Check sheet for the modelled part. Datum: model origin and axes. Units: mm. Coordinates: 2 decimals unless noted, no trailing zeros. Use CSV: the item, a comma, the result in double quotes.
```python
from build123d import *

# Parameters (mm, degrees)
SKETCH_1_R          = 1
EXTRUDE_1_DEPTH     = 2
SKETCH_2_R          = 1
CUT_EXTRUDE_1_DEPTH = 10
SKETCH_3_R          = 1.5
CUT_EXTRUDE_2_DEPTH = 10


with BuildPart() as part:
    # 草圖1 → 填料-伸長1 (new body)
    with BuildSketch(Plane.XY):
        with BuildLine():
            Line((23.861531606, 13.243524775), (25.861531606, 13.243524775))
            ThreePointArc((25.861531606, 13.243524775), (26.568638387, 13.536417994), (26.861531606, 14.243524775))
            Line((26.861531606, 14.243524775), (26.861531606, 16.243524775))
            Line((26.861531606, 16.243524775), (80.861531606, 16.243524775))
            Line((80.861531606, 16.243524775), (81.861531606, 16.243524775))
            Line((81.861531606, 16.243524775), (81.861531606, 15.243524775))
            Line((81.861531606, 15.243524775), (81.861531606, -7.006475225))
            Line((81.861531606, -7.006475225), (79.861531606, -7.006475225))
            ThreePointArc((79.861531606, -7.006475225), (79.154424825, -7.299368444), (78.861531606, -8.006475225))
            Line((78.861531606, -8.006475225), (78.861531606, -10.006475225))
            ThreePointArc((78.861531606, -10.006475225), (79.154424825, -10.713582006), (79.861531606, -11.006475225))
            Line((79.861531606, -11.006475225), (81.861531606, -11.006475225))
            Line((81.861531606, -11.006475225), (81.861531606, -39.006475225))
            Line((81.861531606, -39.006475225), (81.861531606, -40.006475225))
            Line((81.861531606, -40.006475225), (80.861531606, -40.006475225))
            Line((80.861531606, -40.006475225), (61.861531606, -40.006475225))
            Line((61.861531606, -40.006475225), (61.861531606, -38.006475225))
            ThreePointArc((61.861531606, -38.006475225), (61.568638387, -37.299368444), (60.861531606, -37.006475225))
            Line((60.861531606, -37.006475225), (58.861531606, -37.006475225))
            ThreePointArc((58.861531606, -37.006475225), (58.154424825, -37.299368444), (57.861531606, -38.006475225))
            Line((57.861531606, -38.006475225), (57.861531606, -40.006475225))
            Line((57.861531606, -40.006475225), (-8.138468394, -40.006475225))
            Line((-8.138468394, -40.006475225), (-8.138468394, -38.006475225))
            ThreePointArc((-8.138468394, -38.006475225), (-8.431361613, -37.299368444), (-9.138468394, -37.006475225))
            Line((-9.138468394, -37.006475225), (-11.138468394, -37.006475225))
            ThreePointArc((-11.138468394, -37.006475225), (-11.845575175, -37.299368444), (-12.138468394, -38.006475225))
            Line((-12.138468394, -38.006475225), (-12.138468394, -40.006475225))
            Line((-12.138468394, -40.006475225), (-31.138468394, -40.006475225))
            Line((-31.138468394, -40.006475225), (-32.138468394, -40.006475225))
            Line((-32.138468394, -40.006475225), (-32.138468394, -39.006475225))
            Line((-32.138468394, -39.006475225), (-32.138468394, -11.006475225))
            Line((-32.138468394, -11.006475225), (-30.138468394, -11.006475225))
            ThreePointArc((-30.138468394, -11.006475225), (-29.431361613, -10.713582006), (-29.138468394, -10.006475225))
            Line((-29.138468394, -10.006475225), (-29.138468394, -8.006475225))
            ThreePointArc((-29.138468394, -8.006475225), (-29.431361613, -7.299368444), (-30.138468394, -7.006475225))
            Line((-30.138468394, -7.006475225), (-32.138468394, -7.006475225))
            Line((-32.138468394, -7.006475225), (-32.138468394, 15.243524775))
            Line((-32.138468394, 15.243524775), (-32.138468394, 16.243524775))
            Line((-32.138468394, 16.243524775), (-31.138468394, 16.243524775))
            Line((-31.138468394, 16.243524775), (22.861531606, 16.243524775))
            Line((22.861531606, 16.243524775), (22.861531606, 14.243524775))
            ThreePointArc((22.861531606, 14.243524775), (23.154424825, 13.536417994), (23.861531606, 13.243524775))
        make_face()
        with Locations((55.861531606, -36.006475225)):
            Circle(SKETCH_1_R, mode=Mode.SUBTRACT)
        with Locations((77.861531606, -5.006475225)):
            Circle(SKETCH_1_R, mode=Mode.SUBTRACT)
        with Locations((-6.138468394, -36.006475225)):
            Circle(SKETCH_1_R, mode=Mode.SUBTRACT)
        with Locations((28.861531606, 12.243524775)):
            Circle(SKETCH_1_R, mode=Mode.SUBTRACT)
        with Locations((20.861531606, 12.243524775)):
            Circle(SKETCH_1_R, mode=Mode.SUBTRACT)
        with Locations((-28.138468394, -5.006475225)):
            Circle(SKETCH_1_R, mode=Mode.SUBTRACT)
        with Locations((-28.138468394, -13.006475225)):
            Circle(SKETCH_1_R, mode=Mode.SUBTRACT)
        with Locations((77.861531606, -13.006475225)):
            Circle(SKETCH_1_R, mode=Mode.SUBTRACT)
        with Locations((-14.138468394, -36.006475225)):
            Circle(SKETCH_1_R, mode=Mode.SUBTRACT)
        with Locations((63.861531606, -36.006475225)):
            Circle(SKETCH_1_R, mode=Mode.SUBTRACT)
    extrude(amount=EXTRUDE_1_DEPTH)

    # 草圖2 → 除料-伸長1 (cut)
    with BuildSketch(Plane.XY.offset(2)):
        with Locations((7.861531606, -21.006475225)):
            Circle(SKETCH_2_R)
        with Locations((41.861531606, -21.006475225)):
            Circle(SKETCH_2_R)
    extrude(amount=-CUT_EXTRUDE_1_DEPTH, mode=Mode.SUBTRACT)

    # 草圖3 → 除料-伸長2 (cut)
    with BuildSketch(Plane.XY.offset(2)):
        with Locations((-20.138468394, -36.006475225)):
            Circle(SKETCH_3_R)
        with Locations((-20.138468394, 12.243524775)):
            Circle(SKETCH_3_R)
        with Locations(Location((69.861531606, 12.243524775, 0), (0, 0, 180))):
            Circle(SKETCH_3_R)
        with Locations(Location((69.861531606, -36.006475225, 0), (0, 0, 180))):
            Circle(SKETCH_3_R)
    extrude(amount=-CUT_EXTRUDE_2_DEPTH, mode=Mode.SUBTRACT)


solid = part.part
```
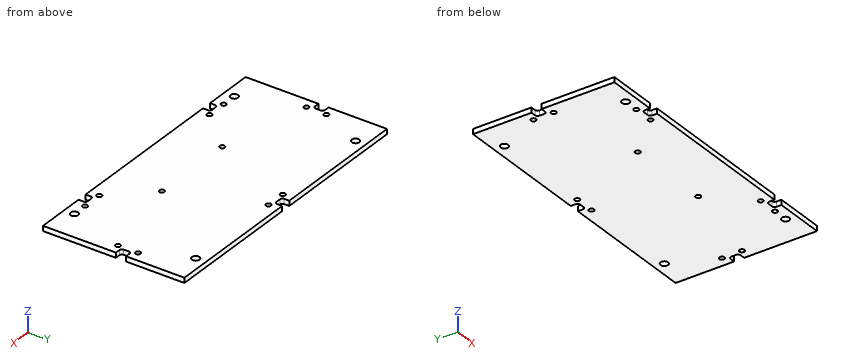
1) Cross-section at A-A on z = 0.55. Give the number of separate pieces and of enclosed holes in the cut face, and give its area (3 significant figures).
Answer below:
separate pieces,"1"
enclosed holes,"16"
area,"6,290 mm²"
2) Thickness scan on line 1 along X through (y, z) = (-21, 0.75); line 2 along X through (y, z) = (11, 1.15); line 3 along Y through (x, z) = (21, 1.95). Record the ranges inside material, lowest first. Write a range as from..to.
Answer below:
line 1,"x = -32.14..6.86, 8.86..40.86, 42.86..81.86"
line 2,"x = -32.14..-20.98, -19.3..69.02, 70.7..81.86"
line 3,"y = -40.01..11.25, 13.23..16.24"
3) Go/stop test with flat-tipped pins: pin 1 Ø1.6 at (x, y) = (41.86, -21.01) entering from +Z; pin 2 Ø0.6 at (y, z) = (-9.5, 1) entering from +X. Record where each tip stops, or that it passes through.
Answer below:
pin 1,"passes through"
pin 2,"stops at x = 78.86"
